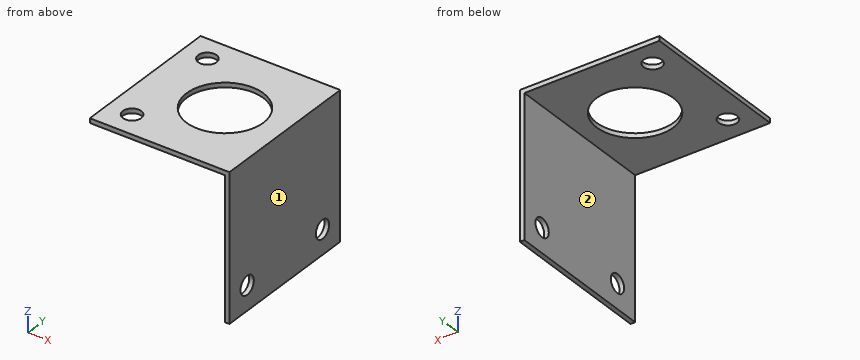
Autodesk Inventor part; units mm, degrees
ref_plane "YZ Plane" through (0, 0, 0) normal (1, 0, 0) x (0, 1, 0)
ref_plane "XZ Plane" through (0, 0, 0) normal (0, 1, 0) x (-1, 0, 0)
ref_plane "XY Plane" through (0, 0, 0) normal (0, 0, 1) x (1, 0, 0)
sketch "Esboço1" plane through (0, 0, 0) normal (0, 0, 1) x (1, 0, 0)
  circle A0 centre (0, 0) radius 12.5
  line L0 (0, 0) -> (18, 0) construction
  line L1 (0, 0) -> (-26, 0) construction
  line L2 (0, 0) -> (0, 25) construction
  line L3 (0, 0) -> (0, -25) construction
  line L4 (-26, 25) -> (18, 25)
  line L5 (18, 25) -> (18, -25)
  line L6 (18, -25) -> (-26, -25)
  line L7 (-26, -25) -> (-26, 25)
  line L8 (-26, 25) -> (-18, 25) construction
  line L9 (-18, 25) -> (-18, 17) construction
  circle A1 centre (-18, 17) radius 3
  line L10 (-26, -25) -> (-18, -25) construction
  line L11 (-18, -25) -> (-18, -17) construction
  circle A2 centre (-18, -17) radius 3
  dimension "d0" = 25
  dimension "d1" = 18
  dimension "d2" = 26
  dimension "d3" = 25
  dimension "d4" = 25
  dimension "d5" = 8
  dimension "d6" = 8
  dimension "d7" = 6
  dimension "d8" = 8
  dimension "d9" = 8
  dimension "d10" = 6
extrude "Extrusão1" add sketch "Esboço1" along normal blind 1.5
sketch "Esboço2" plane through (18, -25, 0) normal (1, 0, 0) x (0, 0, -1)
  line L0 (-1.5, 50) -> (46, 50)
  line L1 (46, 50) -> (46, 0)
  line L2 (46, 0) -> (-1.5, 0)
  line L3 (-1.5, 0) -> (-1.5, 50)
  line L4 (46, 50) -> (38, 50) construction
  line L5 (38, 50) -> (38, 42) construction
  circle A0 centre (38, 42) radius 3
  line L6 (46, 0) -> (38, 0) construction
  line L7 (38, 0) -> (38, 8) construction
  circle A1 centre (38, 8) radius 3
  point P0 (0, 25)
  dimension "d13" = 47.5
  dimension "d14" = 50
  dimension "d15" = 8
  dimension "d16" = 8
  dimension "d17" = 6
  dimension "d18" = 8
  dimension "d19" = 8
  dimension "d20" = 6
extrude "Extrusão2" add sketch "Esboço2" along normal blind 1.5
properties part number "ks dianteiro F" material "Aço cromado"
Build history of the part. All positions in model axes, mm. Face numbers are marked on the shaded views. A direction names the side the tool comes from. Round coordinates to 2 decimals unless told otherwise and drop trailing zeros. Order: outer loops, then holes, each group sorted by start corner. A loop starts at its lowest first (then second) coordinate and runs counter-clockwise, first axis right, second up. Notation, with made-up numbers: (21, -26.5) - (63, -26.5) arc R21 ccw to (63, 10.5) - close; hole circle Ø4 at (54, 47). An arc over 180 degrees is marked (long way). Use a Markdown table: item, result.
1) Tool access for the marked faces 1 and 2: list every direction of +Z, -Z, +X, -X, +Y, -Y with a clear straight run to the whole face (end or side of a thin tool).
Recorded:
| item | result |
|---|---|
| face 1 | +Z, -Z, +X, +Y, -Y |
| face 2 | -Z, -X, +Y, -Y |
2) Flat gauge pins, fed straight in: pin 1 Ø9.5 at (x, y) = (-18, -17) entering from +Z; pin 2 Ø5 at (x, y) = (-18, 17) entering from -Z; pin 3 Ø6 at (x, y) = (14, 8.5) entering from -Z. Where does each tip first touch, or does it go through?
Recorded:
| item | result |
|---|---|
| pin 1 | stops at z = 1.5 |
| pin 2 | passes through |
| pin 3 | stops at z = 0 |
3) Saw through at C-C on x = 0. Write the cut outline in (y, z), and give its area (3 significant figures).
Recorded:
| item | result |
|---|---|
| outline | (-25, 0) - (-12.5, 0) - (-12.5, 1.5) - (-25, 1.5) - close; (12.5, 0) - (25, 0) - (25, 1.5) - (12.5, 1.5) - close |
| area | 37.5 mm² |
4) Saw through at B-B on z = -38. Write the cut outline in (x, y).
Recorded:
| item | result |
|---|---|
| outline | (18, -25) - (19.5, -25) - (19.5, -20) - (18, -20) - close; (18, -14) - (19.5, -14) - (19.5, 14) - (18, 14) - close; (18, 20) - (19.5, 20) - (19.5, 25) - (18, 25) - close |
5) Saw through at A-A on y = 0. Write the cut outline in (x, z).
Recorded:
| item | result |
|---|---|
| outline | (-26, 0) - (-12.5, 0) - (-12.5, 1.5) - (-26, 1.5) - close; (12.5, 0) - (18, 0) - (18, -46) - (19.5, -46) - (19.5, 1.5) - (12.5, 1.5) - close |
6) Wall check: L1, parallel to Y at x = 19.1, z = -38; L2, parallel to X at y = 11.5, z = -0.5; L3, parallel to Z at x = -19.5, y = -12. Give the ranges that are in metal, low to high.
Recorded:
| item | result |
|---|---|
| L1 | y = -25 to -20, -14 to 14, 20 to 25 |
| L2 | x = 18 to 19.5 |
| L3 | z = 0 to 1.5 |
7) Saw through at D-D on y = -15. Write the cut outline in (x, z).
Recorded:
| item | result |
|---|---|
| outline | (-26, 0) - (-20.24, 0) - (-20.24, 1.5) - (-26, 1.5) - close; (-15.76, 0) - (18, 0) - (18, -35.76) - (19.5, -35.76) - (19.5, 1.5) - (-15.76, 1.5) - close; (18, -46) - (19.5, -46) - (19.5, -40.24) - (18, -40.24) - close |
